Check sheet for the modelled part. Datum: model origin and axes. Units: mm. Face numbers are marked on the shaded views. A direction names the side the tool comes from. Round coordinates to 2 decimals unless told otherwise and drop trailing zeros. Order: outer loops, then holes, each group sorted by start corner. A loop starts at its lowest first (then second) coordinate and runs counter-clockwise, first axis right, second up.
Autodesk Inventor part; units mm, degrees
ref_plane "Начальная плоскость" through (0, 0, -23) normal (0, 0, 1) x (1, 0, 0)
ref_plane "Конечная плоскость" through (0, 0, 278) normal (0, 0, 1) x (1, 0, 0)
ref_plane "РабПлоскость8" through (23, -46.6496, 278) normal (0, 0, 1) x (1, 0, 0)
ref_plane "Начальная плоскость" through (0, 0, -23) normal (0, 0, 1) x (1, 0, 0)
ref_plane "Конечная плоскость" through (0, 0, 278) normal (0, 0, 1) x (1, 0, 0)
sketch "Эскиз" plane through (0, 0, 0) normal (0, 0, 1) x (1, 0, 0)
  line L0 (46, -50) -> (0, -50)
  line L1 (46, -50) -> (46, -46.6496)
  line L2 (43.2392, -43.6591) -> (10.9418, -41.0753)
  line L3 (4.5, -34.0976) -> (4.5, 34.0976)
  line L4 (43.2392, 43.6591) -> (10.9418, 41.0753)
  line L5 (46, 46.6496) -> (46, 50)
  line L6 (0, 50) -> (46, 50)
  line L7 (0, -50) -> (0, 50)
  arc A0 (4.5, -34.0976) -> (10.9418, -41.0753) centre (11.5, -34.0976) ccw
  arc A1 (10.9418, 41.0753) -> (4.5, 34.0976) centre (11.5, 34.0976) ccw
  arc A2 (46, -46.6496) -> (43.2392, -43.6591) centre (43, -46.6496) ccw
  arc A3 (43.2392, 43.6591) -> (46, 46.6496) centre (43, 46.6496) ccw
  line L8 (0, 70) -> (0, -70) construction
  line L9 (-9.3169, 0) -> (55.9016, 0) construction
  point P0 (46, -43.88)
  point P1 (4.5, -40.56)
  point P2 (4.5, 40.56)
  point P3 (46, 43.88)
  dimension "d3" = 46
  dimension "d5" = 4.5
  dimension "d7" = 100
  dimension "d9" = 9.44
  dimension "d11" = 9.44
  dimension "d13" = 6.12
  dimension "d15" = 6.12
  dimension "d22" = 7
  dimension "d23" = 3
  dimension "d24" = 50
  dimension "d25" = 0
extrude "Тело" add sketch "Эскиз" along normal up to surface (301 mm away) from surface at -23
sketch "Sketch3" plane through (0, 0, 0) normal (0, 0, 1) x (1, 0, 0)
  line L0 (0, 0) -> (10, 0)
ref_plane "Work Plane7" through (0, 0, 0) normal (0, -1, 0) x (1, 0, 0)
sketch "Sketch4" plane through (0, 0, 0) normal (0, -1, 0) x (1, 0, 0)
  line L0 (-2, -23) -> (12, -23)
  line L1 (-2, 278) -> (12, 278)
  dimension "d29" = 301
ref_plane "РабПлоскость8" through (23, -46.6496, 278) normal (0, 0, 1) x (1, 0, 0)
split "Разделение1" plane through (23, -46.6496, 278) removes the side toward (0, 0, 1)
ref_plane "РабПлоскость9" through (-427, -46.6496, -23) normal (0, 0, -1) x (-1, 0, 0)
split "Разделение2" plane through (-427, -46.6496, -23) removes the side toward (0, 0, -1)
equation "\"d3\" = b"
equation "\"d7\" = ParH"
equation "\"d22\" = R"
equation "\"d23\" = R1"
equation "\"d24\" = 0.5 * d7"
equation "\"d16\" = G_L"
equation "\"R1\" = 3"
equation "\"R\" = 7"
equation "\"t1\" = 4.5"
equation "\"t2\" = 7.6"
equation "\"ParH\" = 100"
equation "\"b\" = 46"
equation "\"msp_x1\" = 0.04 * b"
equation "\"msp_x2\" = -0.08 * t1 + 0.04 * b"
equation "\"G_L\" = d29"
equation "\"ex\" = 0"
equation "\"G_OFFSET_START\" = 23"
equation "\"G_OFFSET_END\" = 23"
equation "\"d26\" = -G_OFFSET_START"
equation "\"d27\" = G_OFFSET_END + B_L"
equation "\"B_L\" = 255"
properties part number "Швеллер 10U-301 ГОСТ 8240-97" material "Сталь, мягкая, сварочная"
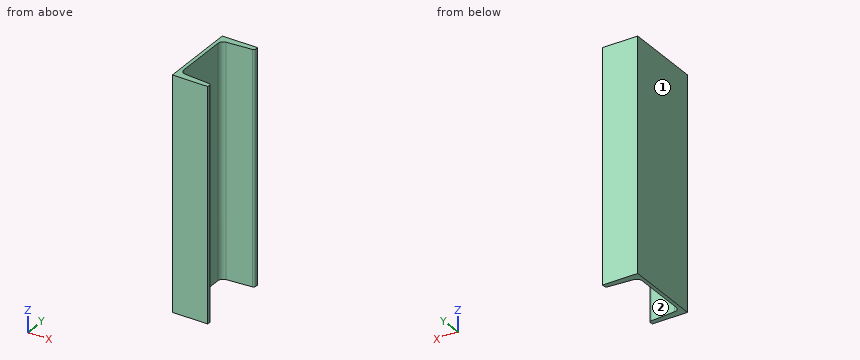
Item 1: Sectioned sample at C-C (x = 38.5). Record the cut outline in (y, z).
Answer:
outline: (-50, -23) - (-43.28, -23) - (-43.28, 278) - (-50, 278) - close; (43.28, -23) - (50, -23) - (50, 278) - (43.28, 278) - close
Item 2: Access from +Z, -Z, +X, -X, +Y, -Y to the whole of each face (thin tool, end or side, straight path). Record for the marked faces 1 and 2.
Answer:
face 1: +Z, -Z, -X, +Y, -Y
face 2: +Z, -Z, +X
Item 3: Sectioned sample at A-A (x = 15). Record the cut outline in (y, z), and give its area (3 significant figures).
Answer:
outline: (-50, -23) - (-41.4, -23) - (-41.4, 278) - (-50, 278) - close; (41.4, -23) - (50, -23) - (50, 278) - (41.4, 278) - close
area: 5,180 mm2
Item 4: Sectioned sample at D-D (y = 19). Record the cut outline in (x, z).
Answer:
outline: (0, -23) - (4.5, -23) - (4.5, 278) - (0, 278) - close
Item 5: Go/stop test with flat-tipped pins: P1, Ø5, axis at y = -37.5, z = 143, coming from the +X side; P2, Ø2, axis at y = 5.5, z = 23, coming from the +X side. Record where each tip stops, or that it passes through.
Answer:
P1: stops at x = 7.74
P2: stops at x = 4.5
Item 6: Sectioned sample at B-B (z = 250.5). Record the cut outline in (x, y), and give its area (3 significant figures).
Answer:
outline: (0, -50) - (46, -50) - (46, -46.65) arc R3 ccw to (43.24, -43.66) - (10.94, -41.08) arc R7 cw to (4.5, -34.1) - (4.5, 34.1) arc R7 cw to (10.94, 41.08) - (43.24, 43.66) arc R3 ccw to (46, 46.65) - (46, 50) - (0, 50) - close
area: 1,110 mm2
Item 7: Scan lines: line 1 along Y through (x, z) = (10.5, 70); line 2 along Y through (x, z) = (6.5, 29); line 3 along X through (y, z) = (-10.5, 10). Record each from-to range of solid material in increasing order.
Answer:
line 1: y = -50 to -41.03, 41.03 to 50
line 2: y = -50 to -39, 39 to 50
line 3: x = 0 to 4.5
